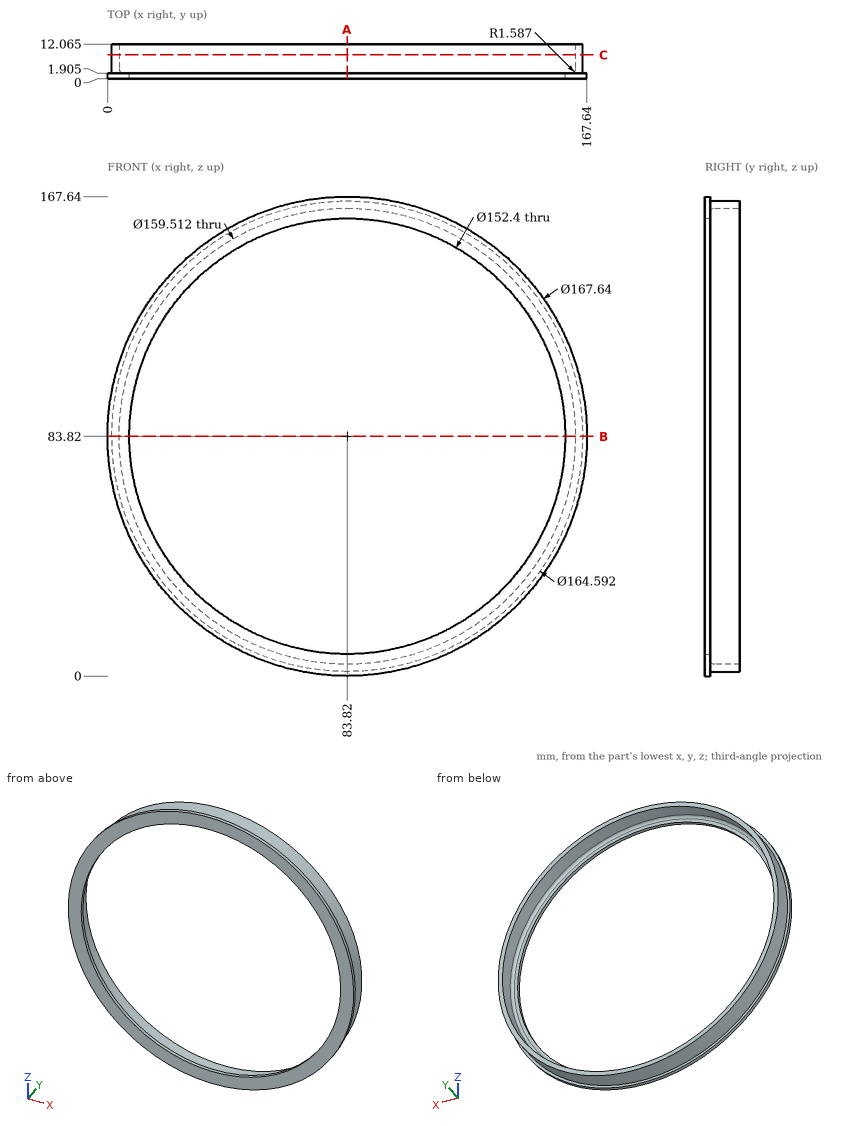
Can you work these out from the drawing? Everything is in mm from the part's minimum corner. Coordinates: 2 decimals unless noted, no trailing zeros. Order: outer loops, then holes, each group sorted by start corner. A loop starts at its lowest first (then second) coordinate and runs counter-clockwise, first axis right, second up. Notation, with made-up numbers: (71.25, -37) -> (93.25, -37) arc R25 cw to (93.25, -9) -> close; hole circle Ø5 at (61, 13.25). An arc over 180 degrees is marked (long way). Use one line per item in the form item = value.
Q1. Imagine slicing it at B-B, the plane z = 83.82. List the corners of the cut face in (x, y) for me (1 decimal).
From the geometry:
outline = (0, 0) -> (7.6, 0) -> (7.6, 1.9) -> (5.7, 1.9) arc R1.6 cw to (4.1, 3.5) -> (4.1, 12.1) -> (1.5, 12.1) -> (1.5, 1.9) -> (0, 1.9) -> close; (160, 0) -> (167.6, 0) -> (167.6, 1.9) -> (166.1, 1.9) -> (166.1, 12.1) -> (163.6, 12.1) -> (163.6, 3.5) arc R1.6 cw to (162, 1.9) -> (160, 1.9) -> close
Q2. Will these pins go through, and if not, where does the flat tip stop? P1, Ø1.5, axis at x = 31, y = 4, coming from the +Z side; P2, Ø3, axis at x = 67, y = 4, coming from the -Z side; P3, Ø4, axis at x = 124, y = 4.5, coming from the -Z side.
From the geometry:
P1 = 147.55
P2 = 2.96
P3 = 10.92
Q3. I need wall thicknesses on L1, parallel to X at y = 1.5, z = 83.5; L2, parallel to X at y = 1.25, z = 98.5 (1 decimal); L3, parallel to Y at x = 18, z = 126.5. Which ranges of each line are inside material? Lowest first, please.
From the geometry:
L1 = 0 to 7.62, 160.02 to 167.64
L2 = 1.3 to 9, 158.6 to 166.3
L3 = 0 to 1.93
Q4. Imagine slicing it at A-A, the plane x = 83.82. List the corners of the cut face in (y, z) for me (1 decimal).
From the geometry:
outline = (0, 0) -> (1.9, 0) -> (1.9, 1.5) -> (12.1, 1.5) -> (12.1, 4.1) -> (3.5, 4.1) arc R1.6 cw to (1.9, 5.7) -> (1.9, 7.6) -> (0, 7.6) -> close; (0, 160) -> (1.9, 160) -> (1.9, 162) arc R1.6 cw to (3.5, 163.6) -> (12.1, 163.6) -> (12.1, 166.1) -> (1.9, 166.1) -> (1.9, 167.6) -> (0, 167.6) -> close
Q5. Imagine slicing it at C-C, the plane y = 8.25. List the corners of the cut face in (x, z) for me (1 decimal).
From the geometry:
outline = circle Ø164.6 at (83.8, 83.8); hole circle Ø159.5 at (83.8, 83.8)
